from build123d import *

# Parameters (mm, degrees)
F1_DEPTH = 5


with BuildPart() as f1:
    # F0 (on Front) → F1 (new body)
    with BuildSketch(Plane.XZ):
        Polygon((0, 5), (0, 0), (50, 0), (50, 5), (30.84, 5), (29.83, 5), (29.27, 5), (28.26, 5), (27.7, 5), (26.69, 5), (26.13, 5), (25.12, 5), (24.56, 5), (23.55, 5), (22.99, 5), (21.98, 5), (21.42, 5), (20.41, 5), (19.85, 5), (18.84, 5), (18.28, 5), (17.27, 5), (16.71, 5), (15.7, 5), (15.14, 5), (14.13, 5), (13.57, 5), (12.56, 5), (12, 5), (10.99, 5), (10.43, 5), (9.42, 5), (8.86, 5), (7.85, 5), (7.29, 5), (6.28, 5), (5.72, 5), (4.71, 5), (4.15, 5), (3.14, 5), (2.58, 5), (1.57, 5), (1.01, 5), align=None)
        Polygon((0.19396, 6.1), (0, 5), (1.01, 5), (0.81604, 6.1), align=None)
        Polygon((29.83, 5), (30.84, 5), (30.64604, 6.1), (30.02396, 6.1), align=None)
        Polygon((1.76396, 6.1), (1.57, 5), (2.58, 5), (2.38604, 6.1), align=None)
        Polygon((28.26, 5), (29.27, 5), (29.07604, 6.1), (28.45396, 6.1), align=None)
        Polygon((3.33396, 6.1), (3.14, 5), (4.15, 5), (3.95604, 6.1), align=None)
        Polygon((26.69, 5), (27.7, 5), (27.50604, 6.1), (26.88396, 6.1), align=None)
        Polygon((4.90396, 6.1), (4.71, 5), (5.72, 5), (5.52604, 6.1), align=None)
        Polygon((25.12, 5), (26.13, 5), (25.93604, 6.1), (25.31396, 6.1), align=None)
        Polygon((6.47396, 6.1), (6.28, 5), (7.29, 5), (7.09604, 6.1), align=None)
        Polygon((23.55, 5), (24.56, 5), (24.36604, 6.1), (23.74396, 6.1), align=None)
        Polygon((8.04396, 6.1), (7.85, 5), (8.86, 5), (8.66604, 6.1), align=None)
        Polygon((21.98, 5), (22.99, 5), (22.79604, 6.1), (22.17396, 6.1), align=None)
        Polygon((9.61396, 6.1), (9.42, 5), (10.43, 5), (10.23604, 6.1), align=None)
        Polygon((20.41, 5), (21.42, 5), (21.22604, 6.1), (20.60396, 6.1), align=None)
        Polygon((11.18396, 6.1), (10.99, 5), (12, 5), (11.80604, 6.1), align=None)
        Polygon((18.84, 5), (19.85, 5), (19.65604, 6.1), (19.03396, 6.1), align=None)
        Polygon((12.75396, 6.1), (12.56, 5), (13.57, 5), (13.37604, 6.1), align=None)
        Polygon((17.27, 5), (18.28, 5), (18.08604, 6.1), (17.46396, 6.1), align=None)
        Polygon((14.32396, 6.1), (14.13, 5), (15.14, 5), (14.94604, 6.1), align=None)
        Polygon((15.7, 5), (16.71, 5), (16.51604, 6.1), (15.89396, 6.1), align=None)
    extrude(amount=F1_DEPTH)


solid = f1.part
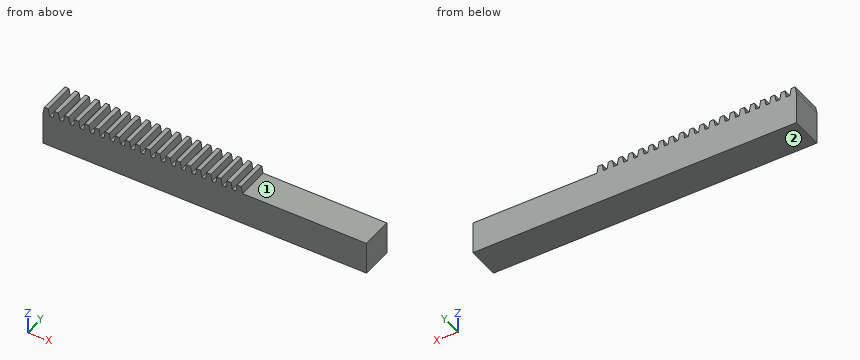
Verification items for the finished model (mm, model axes). Face numbers are marked on the shaded views. A direction names the side the tool comes from. Give positions to 0.01 mm unless a question says otherwise; leave off trailing zeros. Write each loop counter-clockwise with the first axis right and the second up, starting at its lowest first coordinate (ties: lowest second). Pieces come first, ordered by that corner, then holes.
(1) Cross-section at B-B (x = 38.5). Enter the section's corners in (y, z).
(2) Access from +Z, -Z, +X, -X, +Y, -Y to the whole of each face (thin tool, end or side, straight path). Record for the marked faces 1 and 2.
(3) Gauge pin test, flat end, axial feed: pin 1 (2.5 mm diameter, centred on x = 41.5, y = -3, fed in from +Z). Record the tip position at first contact, or that the pin passes through.
(4) Cross-section at A-A (z = 5.5). State how many separate pieces and enclosed holes the cut face has, plus the area to 3 significant figures.
(5) Material ranges on line 1 (Z direction, x = 32, y = -3.6), recorded low to high.
Worked out:
1. outline: (-5, 0) - (0, 0) - (0, 5) - (-5, 5) - close
2. face 1: +Z, +X, +Y, -Y
2. face 2: -Z, +X, -X, +Y, -Y
3. pin 1: stops at z = 5
4. separate pieces: 20
4. enclosed holes: 0
4. area: 83.4 mm2
5. line 1: z = 0 to 5
